Model file for the job. Use its own axes, mm. A direction names the side the tool comes from. Give positions to 0.01 mm unless a question says otherwise; leave off trailing zeros. Loops run counter-clockwise (first coordinate to the right, second up) from the corner with the lowest first, then second, coordinate; pieces in that order, holes last. Notation, with made-up numbers: M 16.25,74.25 L 41.25,74.25 A12 ccw 41.25,96.25 Z; hole C -11,4.25 d3. An arc over 180 degrees is marked long. Use CSV: the item, a comma, the result in double quotes. Start each with the question number.
(1) Two-plate mould, pull along X, no slides. Class faces 4 (the face through (-2.15, 0.05, -6)), 5 (the face through (-0.8, 1.4, -9.88)), 6 (the face through (-3.233, -1.341, -7.975)): pulls with the +X half, pulls with the -X half, needs draft (parallel to the pull), parting line crosses it, or undercut.
(2) Slice it at B-B on z = -5. List the corners of the cut face in (x, y), and give its area (3 significant figures).
(3) Slice it at C-C on z = -7.25. List the corners of the cut face in (x, y).
(4) Slice it at A-A on y = 0. List the corners of the cut face in (x, z), and give its area (3 significant figures).
(5) Tool access for faces 1 (the face through (0, 0, 0)), 2 (the face through (0, -2, -3)), 3 (the face through (-0.82, -1.39, -9.88)): list every direction of +Z, -Z, +X, -X, +Y, -Y with a clear straight run to the whole face (end or side of a thin tool).
(6) Wall check: line 1 along Y through (x, z) = (-1, -5.5); line 2 along Z through (x, y) = (2.75, -1.25). Give the ranges that are in metal, low to high. Write a range as from..to.
(7) Flat gauge pins, fed straight in: P1, Ø3, axis at y = -1.5, z = -3.5, coming from the +X side; P2, Ø3, axis at y = 2, z = -2.5, coming from the +X side; P3, Ø1.5, axis at x = 2.5, z = -4, coming from the -Y side. Where does each tip first touch, or does it go through?
```python
from build123d import *

# Parameters (mm, degrees)
SKETCH1_R           = 2
EXTRUDE1_DEPTH      = 6
CUT_SWEEP1_PITCH    = 0.7
SKETCH6_R           = 3.5
EXTRUDE2_DEPTH      = 4
CUT_EXTRUDE1_DEPTH  = 2.25
CHAMFER1_SIZE       = 0.21
SKETCH12_R          = 2
BOSS_EXTRUDE1_DEPTH = 6
CHAMFER2_SIZE       = 0.5
CHAMFER2_SIZE_2     = 0.866025404


with BuildPart() as part:
    # Sketch1 → Extrude1 (new body)
    with BuildSketch(Plane.XY):
        Circle(SKETCH1_R)
    extrude(amount=-EXTRUDE1_DEPTH)

    # Cut-Sweep1: the profile of Sketch3 profile screwed along a right-hand helix of 9.571429 turns, 6 arcs to a turn; built about Z, then put on its axis
    cut_sweep1_z = Axis((0, 0, 0), (0, 0, 1))
    cut_sweep1_corners = [(2.0003, 0, -0.612673205), (1.545336663, 0, -0.35), (1.545336663, 0, -0.2625), (2.0003, 0, 0.000173205)]
    with BuildLine(mode=Mode.PRIVATE) as cut_sweep1_profile:
        Line(cut_sweep1_corners[0], cut_sweep1_corners[1])
        Line(cut_sweep1_corners[1], cut_sweep1_corners[2])
        Line(cut_sweep1_corners[2], cut_sweep1_corners[3])
        Line(cut_sweep1_corners[3], cut_sweep1_corners[0])
    cut_sweep1_cap = Face(cut_sweep1_profile.wire())
    cut_sweep1_turn_angles = [0, 30, 60, 90, 120, 150, 180, 210, 240, 270, 300, 330, 360]
    cut_sweep1_turn_weights = [1, 0.8660254037844387, 1, 0.8660254037844387, 1, 0.8660254037844387, 1, 0.8660254037844387, 1, 0.8660254037844387, 1, 0.8660254037844387, 1]
    cut_sweep1_turn_rails = [Edge.make_bspline([Vector(p[0], p[1], 0).rotate(cut_sweep1_z, cut_sweep1_turn_angles[k]) / cut_sweep1_turn_weights[k] + Vector(0, 0, p[2] + CUT_SWEEP1_PITCH * cut_sweep1_turn_angles[k] / 360) for k in range(13)], [0, 0, 0, 1, 1, 2, 2, 3, 3, 4, 4, 5, 5, 6, 6, 6], 2, cut_sweep1_turn_weights) for p in cut_sweep1_corners]
    cut_sweep1_turn_sides = [Face.make_surface_from_curves(cut_sweep1_turn_rails[p[0]], cut_sweep1_turn_rails[p[1]]) for p in [(0, 1), (1, 2), (2, 3), (3, 0)]]
    cut_sweep1_last_angles = [3240, 3270, 3300, 3330, 3360, 3390, 3420, 3432.857142857, 3445.714285714]
    cut_sweep1_last_weights = [1, 0.8660254037844387, 1, 0.8660254037844387, 1, 0.8660254037844387, 1, 0.9749279121818499, 1]
    cut_sweep1_last_rails = [Edge.make_bspline([Vector(p[0], p[1], 0).rotate(cut_sweep1_z, cut_sweep1_last_angles[k]) / cut_sweep1_last_weights[k] + Vector(0, 0, p[2] + CUT_SWEEP1_PITCH * cut_sweep1_last_angles[k] / 360) for k in range(9)], [0, 0, 0, 1, 1, 2, 2, 3, 3, 4, 4, 4], 2, cut_sweep1_last_weights) for p in cut_sweep1_corners]
    cut_sweep1_last_sides = [Face.make_surface_from_curves(cut_sweep1_last_rails[p[0]], cut_sweep1_last_rails[p[1]]) for p in [(0, 1), (1, 2), (2, 3), (3, 0)]]
    cut_sweep1 = Plane(origin=(0, 0, 0), x_dir=(0, 1, 0), z_dir=(0, 0, -1)) * Solid(Shell([*[p.moved(Location((0, 0, CUT_SWEEP1_PITCH * i))) for i in range(9) for p in cut_sweep1_turn_sides], *cut_sweep1_last_sides, cut_sweep1_cap, cut_sweep1_cap.rotate(cut_sweep1_z, 3445.714285714).moved(Location((0, 0, CUT_SWEEP1_PITCH * 3445.714285714 / 360)))]))
    add(cut_sweep1, mode=Mode.SUBTRACT)

    # Sketch4 → Cut-Revolve1 (revolve, cut)
    with BuildSketch(Plane(origin=(0, 0, 0), x_dir=(0, 0, -1), z_dir=(1, 0, 0)), mode=Mode.PRIVATE) as cut_revolve1_sk:
        Polygon((0.496211411, 2), (0, 1.291336663), (0, 2), align=None)
    revolve(cut_revolve1_sk.sketch.rotate(Axis((0, 0, 0), (0, 0, -1)), 271.401126896), axis=Axis((0, 0, 0), (0, 0, -1)), mode=Mode.SUBTRACT)

    # Sketch6 → Extrude2 (add)
    with BuildSketch(Plane(origin=(0, 0, -6), x_dir=(-1, 0, 0), z_dir=(0, 0, -1))):
        Circle(SKETCH6_R)
    extrude(amount=EXTRUDE2_DEPTH)

    # Sketch7 → Cut-Extrude1 (cut)
    with BuildSketch(Plane(origin=(0, 0, -10), x_dir=(-1, 0, 0), z_dir=(0, 0, -1))):
        Polygon((0, 1.732050808), (-1.5, 0.866025404), (-1.5, -0.866025404), (0, -1.732050808), (1.5, -0.866025404), (1.5, 0.866025404), align=None)
    extrude(amount=-CUT_EXTRUDE1_DEPTH, mode=Mode.SUBTRACT)

    # Cut-Extrude2 cone 1 section (through the dimple's axis) → Cut-Extrude2 (revolve, cut)
    with BuildSketch(Plane(origin=(0, 0, -10), x_dir=(0, 1, 0), z_dir=(1, 0, 0))):
        Polygon((0, 0), (1.732050808, 0), (0, 1.732050808), align=None)
    revolve(axis=Axis((0, 0, -10), (0, 0, 1)), mode=Mode.SUBTRACT)

    # Chamfer1
    chamfer1_edges = [part.edges().sort_by_distance(p)[0] for p in [
        (3.5, 0, -6),
        (3.5, 0, -10),
    ]]
    chamfer(chamfer1_edges, length=CHAMFER1_SIZE)

    # Sketch10 → Revolve1 (revolve)
    with BuildSketch(Plane(origin=(0, 0, 0), x_dir=(0, 0, -1), z_dir=(1, 0, 0)), mode=Mode.PRIVATE) as revolve1_sk:
        Polygon((6, 2), (6, 0), (4.996572875, 0), (5.825, 2), align=None)
    revolve(revolve1_sk.sketch.rotate(Axis((0, 0, -6), (0, 0, 1)), 270), axis=Axis((0, 0, -6), (0, 0, 1)))

    # Sketch12 → Boss-Extrude1 (add)
    with BuildSketch(Plane.XY):
        Circle(SKETCH12_R)
    extrude(amount=-BOSS_EXTRUDE1_DEPTH)

    # Chamfer2
    # the kernel refuses this chamfer: 0.866025404, 0.5 mm, written as the material it takes off along each edge
    with BuildSketch(Plane(origin=(0, 0, 0), x_dir=(1, 0, 0), z_dir=(0, -1, 0))) as chamfer2_piece_1:
        Polygon((2, -CHAMFER2_SIZE), (2 - CHAMFER2_SIZE_2, 0), (2, 0), align=None)
    revolve(axis=Axis((0, 0, 0), (0, 0, 1)), mode=Mode.SUBTRACT)


solid = part.part
```
Reply:
1,face 4,"needs draft"
1,face 5,"undercut"
1,face 6,"parting line crosses it"
2,outline,"C 0,0 d4"
2,area,"12.6 mm^2"
3,outline,"C 0,0 d7"
4,outline,"M -3.5,-9.79 L -3.29,-10 L -1.73,-10 L -1.5,-9.77 L -1.5,-7.75 L 1.5,-7.75 L 1.5,-9.77 L 1.73,-10 L 3.29,-10 L 3.5,-9.79 L 3.5,-6.21 L 3.29,-6 L 2,-6 L 2,-0.5 L 1.13,0 L -1.13,0 L -2,-0.5 L -2,-6 L -3.29,-6 L -3.5,-6.21 Z"
4,area,"44.7 mm^2"
5,face 1,"+Z, +X, -X, +Y, -Y"
5,face 2,"+Z"
5,face 3,"-Z"
6,line 1,"y = -1.73..1.73"
6,line 2,"z = -10..-6"
7,P1,"stops at x = 2"
7,P2,"stops at x = 1.94"
7,P3,"stops at y = -0.97"
